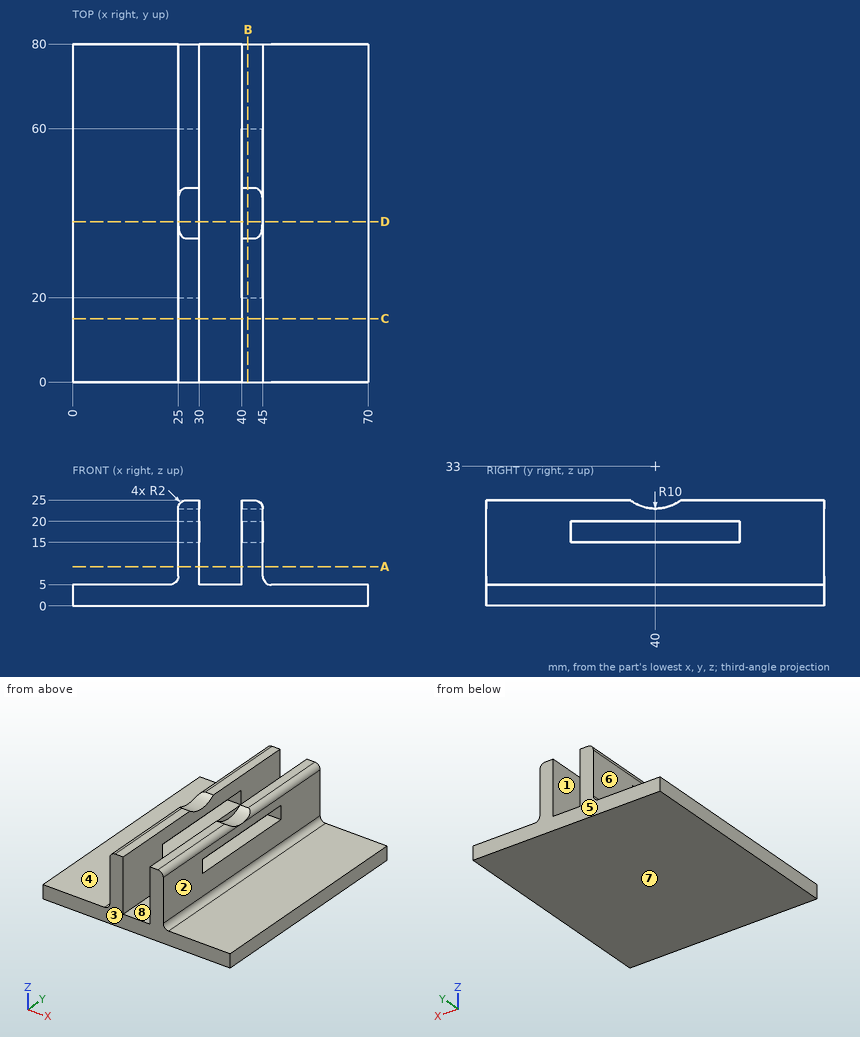
Answer from the drawing. Dimensions are ordinates in mm from the lowest x, y and z of the part. A direction names the side the tool comes from. Give positions to 0.01 mm unless a question says otherwise; leave off trailing zeros. Loops run counter-clockwise (first coordinate to the right, second up) from the corner with the lowest first, then second, coordinate; pieces in that order, holes last.
Item 1: Find the intervals of material crossed by line 1 along X through (y, z) = (75, 21); line 2 along Z through (x, y) = (42, 23); line 3 along Y through (x, z) = (41, 16.75), in increasing order.
Item 2: The part is cut by section A-A (z = 9.25). Write down the section's boundary in (x, y), and give its area (3 significant figures).
Item 3: The part is cut by section B-B (x = 41.5). Write down the section's boundary in (y, z), and give its area (3 significant figures).
Item 4: For the marked faces 1, 2, 3, 4 and 5, determine the directions among +Z, -Z, +X, -X, +Y, -Y from which every point of the face is accessible in a straight line to the end or side of a thin tool.
Item 5: Each of these flat-tipped pins is pushed along its axis until it touches: pin 1 Ø4 at (y, z) = (8.5, 13.5) entering from +X; pin 2 Ø4 at (y, z) = (21, 17.5) entering from -X; pin 3 Ø1.5 at (x, y) = (53, 39) entering from +Z. Where does it stop, or does it pass through?
Item 6: The part is cut by section C-C (y = 15). Write down the section's boundary in (x, z).
Item 7: The part is cut by section D-D (y = 38). Write down the section's boundary in (x, z).
Item 8: The mould has two halves that part along X. Classify the marked faces 6, 7 and 8: released by +X, released by -X, zero draft, split by the parting line, or undercut.
Taken from the geometry:
1. line 1: x = 25 to 30, 40 to 45
1. line 2: z = 0 to 15, 20 to 25
1. line 3: y = 0 to 20, 60 to 80
2. outline: (25, 0) - (30, 0) - (30, 80) - (25, 80) - close; (40, 0) - (45, 0) - (45, 80) - (40, 80) - close
2. area: 800 mm2
3. outline: (0, 0) - (80, 0) - (80, 25) - (46, 25) arc R10 cw to (34, 25) - (0, 25) - close; hole (20, 15) - (60, 15) - (60, 20) - (20, 20) - close
3. area: 1,780 mm2
4. face 1: +Z, +Y, -Y
4. face 2: +Z, +X, +Y, -Y
4. face 3: +Z, -Z, +X, -X, -Y
4. face 4: +Z, -X, +Y, -Y
4. face 5: +Z, -Z, +X, -X, +Y
5. pin 1: stops at x = 45
5. pin 2: stops at x = 25
5. pin 3: stops at z = 5
6. outline: (0, 0) - (70, 0) - (70, 5) - (47, 5) arc R2 cw to (45, 7) - (45, 23) arc R2 ccw to (43, 25) - (40, 25) - (40, 5) - (30, 5) - (30, 25) - (27, 25) arc R2 ccw to (25, 23) - (25, 7) arc R2 cw to (23, 5) - (0, 5) - close
7. outline: (0, 0) - (70, 0) - (70, 5) - (47, 5) arc R2 cw to (45, 7) - (45, 15) - (40, 15) - (40, 5) - (30, 5) - (30, 15) - (25, 15) - (25, 7) arc R2 cw to (23, 5) - (0, 5) - close; (25, 20) - (30, 20) - (30, 23.2) - (25.01, 23.2) arc R2 ccw to (25, 23) - close; (40, 20) - (45, 20) - (45, 23) arc R2 ccw to (44.99, 23.2) - (40, 23.2) - close
8. face 6: released by -X
8. face 7: zero draft
8. face 8: undercut
